Could you check a few things on this drawing? It's one solid part, dimensions in mm from its lowest x, y, z. A direction names the side the tool comes from. Give positions to 0.01 mm unless a question says otherwise; leave off trailing zeros. Loops run counter-clockwise (first coordinate to the right, second up) from the corner with the lowest first, then second, coordinate; pieces in that order, holes last. Notation, with made-up numbers: M 33,-31 L 73,-31 A11 cw 73,-25 Z; hole C -5.5,9 d6. An arc over 180 degrees is marked long. Answer as CSV lines item,"result". Start each with the question number.
Item 1: Will these pins go through, and if not, where does the flat tip stop? P1, Ø5, axis at x = 12.5, z = 7, coming from the -Y side; P2, Ø10, axis at x = 33, y = 10.5, coming from the -Z side; P3, Ø4, axis at y = 7.5, z = 7.5, coming from the +X side; P4, Ø20, axis at x = 20, y = 20, coming from the -Z side.
Item 2: If we mould it in two halves opening along Y, with no side actions, what happens to the marked faces 3, 4 and 5? For each: released by +Y, released by -Y, zero draft, split by the parting line, or undercut.
Item 3: I want a section at A-A on y = 20. List the corners of the cut face in (x, z) for me.
Item 4: For the marked faces 1 and 2, which set-ups out of +Z, -Z, +X, -X, +Y, -Y let a thin tool reach every point of the face, with its end or its side?
Item 5: I want a section at C-C on z = 5.75. List the corners of the cut face in (x, y) for me.
Item 6: If I drill on line 1 along Y through (x, z) = (20, 17.25); line 2 along Z through (x, y) = (28.5, 15); line 3 along X through (y, z) = (20, 13), over which ranges is the centre line in solid material (lowest first)? Write a range as from..to.
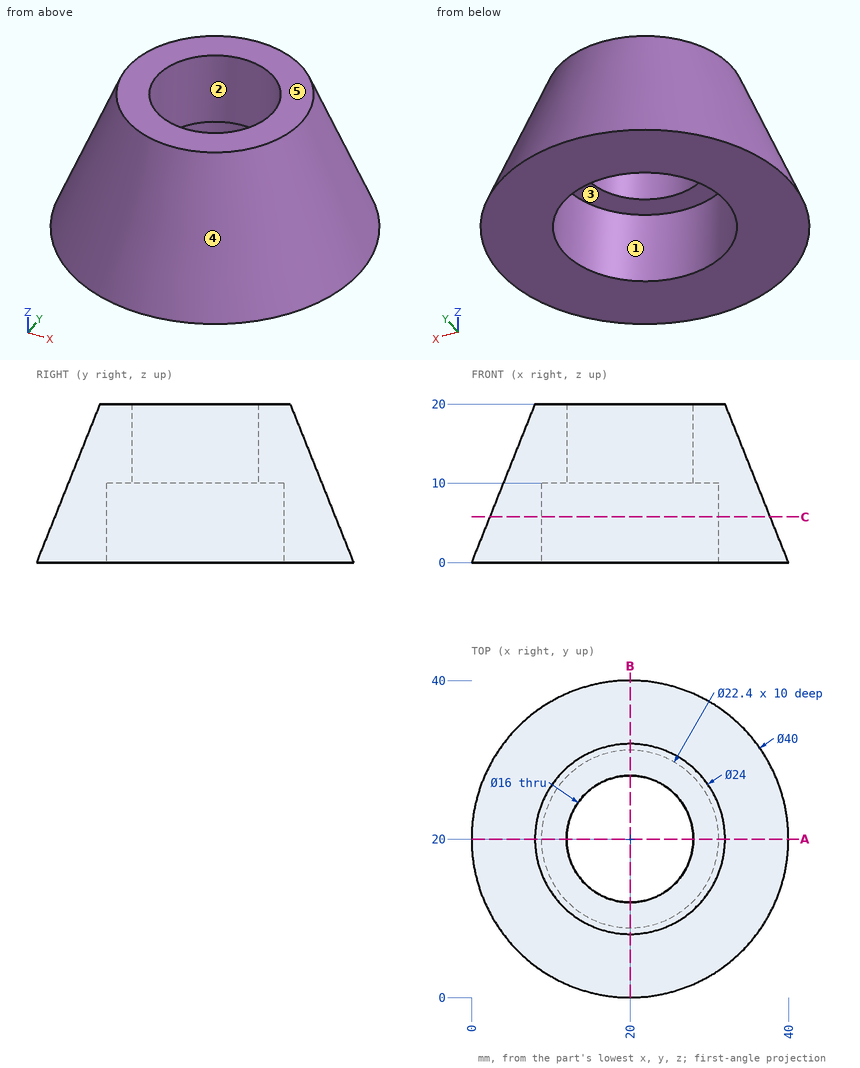
Result:
1,P1,"y = 3.03"
1,P2,"z = 0"
1,P3,"x = 33.67"
1,P4,"z = 10"
2,face 3,"undercut"
2,face 4,"split by the parting line"
2,face 5,"zero draft"
3,outline,"M 0,0 L 8.8,0 L 8.8,10 L 12,10 L 12,20 L 8,20 Z; M 28,10 L 31.2,10 L 31.2,0 L 40,0 L 32,20 L 28,20 Z"
4,face 1,"-Z"
4,face 2,"+Z, -Z"
5,outline,"C 20,20 d35.4; hole C 20,20 d22.4"
6,line 1,"6.9..12, 28..33.1"
6,line 2,"10..20"
6,line 3,"5.2..12, 28..34.8"
